Could you check a few things on this model? Use its own coordinates, in mm. A direction names the side the tool comes from. Coordinates: 2 decimals unless noted, no trailing zeros. Loops run counter-clockwise (first coordinate to the right, second up) from the corner with the lowest first, then second, coordinate; pieces in that order, holes last.
1) Imagine slicing it at C-C on y = 68. Please give me the cut outline in (x, z) (3 decimals), plus the area to 3 significant figures.
2) If I drill on line 1 along X through (y, z) = (61, 18.5) (3 decimals); line 2 along Z through (x, y) = (-19, 66.5); line 3 along Z through (x, y) = (-28, 26), over which ranges is the centre line in solid material (lowest first)?
3) Imagine slicing it at B-B on z = 1.5. Please give me the cut outline in (x, y), plus the area to 3 significant figures.
4) For faces 1 (the face through (-2, 38, 46.253)), 2 (the face through (-3.175, 38, 21)), which set-ups out of +Z, -Z, +X, -X, +Y, -Y let a thin tool reach every point of the face, with its end or its side?
5) Imagine slicing it at D-D on x = -25. Please give me the cut outline in (y, z).
6) Will these pins go through, and if not, where does the flat tip stop? P1, Ø12, axis at x = -7, z = -13.5, coming from the +Y side; P2, Ø21, axis at y = 41, z = 33.5, coming from the -X side (3 decimals); P3, Ø6, axis at y = 35.5, z = -15.5, coming from the -X side; P4, Ø1.5, axis at x = -32.5, y = 48.5, coming from the -Z side.
7) Imagine slicing it at A-A on y = 47.5. Please give me the cut outline in (x, z) (3 decimals), plus the area to 3 significant figures.
```python
from build123d import *

# Parameters (mm, degrees)
BOSS_EXTRUDE2_DEPTH = 76.2
CUT_EXTRUDE3_REACH  = 43.301
CUT_EXTRUDE4_REACH  = 62.908
FILLET1_R           = 5.08
FILLET2_R           = 3.81


with BuildPart() as part:
    # Sketch1 → Boss-Extrude2 (new body)
    with BuildSketch(Plane(origin=(0, 0, 0), x_dir=(1, 0, 0), z_dir=(0, 1, 0))):
        with BuildLine():
            Line((-39.668156778, 23.786852448), (-3.577868638, 2.145454699))
            ThreePointArc((-3.577868638, 2.145454699), (-0.956579917, -0.541770779), (0, -4.171824524))
            Line((0, -4.171824524), (0, -46.2534))
            Line((0, -46.2534), (-3.175, -46.2534))
            Line((-3.175, -46.2534), (-3.175, -4.171824524))
            ThreePointArc((-3.175, -4.171824524), (-3.719260987, -2.106449117), (-5.21068388, -0.577510483))
            Line((-5.21068388, -0.577510483), (-41.300972021, 21.063887265))
            Line((-41.300972021, 21.063887265), (-39.668156778, 23.786852448))
        make_face()
    extrude(amount=BOSS_EXTRUDE2_DEPTH)

    # Sketch2 → Cut-Extrude3 (cut, up to next)
    with BuildSketch(Plane(origin=(0, 0, 0), x_dir=(0, 0, -1), z_dir=(1, 0, 0)), mode=Mode.PRIVATE) as cut_extrude3_sk1:
        Polygon((-46.2534, 53.975), (-18.494383897, 76.2), (-46.2534, 76.2), align=None)
    cut_extrude3_tool1 = extrude(cut_extrude3_sk1.sketch, amount=-CUT_EXTRUDE3_REACH, mode=Mode.PRIVATE) & part.part
    add(cut_extrude3_tool1.solids().sort_by_distance((0, 68.791667, 37.000395))[0], mode=Mode.SUBTRACT)
    # Sketch2 → Cut-Extrude3 (cut, up to next)
    with BuildSketch(Plane(origin=(0, 0, 0), x_dir=(0, 0, -1), z_dir=(1, 0, 0)), mode=Mode.PRIVATE) as cut_extrude3_sk2:
        Polygon((-46.2534, 22.225), (-46.2534, 0), (-18.494383897, 0), align=None)
    cut_extrude3_tool2 = extrude(cut_extrude3_sk2.sketch, amount=-CUT_EXTRUDE3_REACH, mode=Mode.PRIVATE) & part.part
    add(cut_extrude3_tool2.solids().sort_by_distance((0, 7.408333, 37.000395))[0], mode=Mode.SUBTRACT)

    # Sketch4 → Cut-Extrude4 (cut, up to next)
    with BuildSketch(Plane(origin=(0, 0, 0), x_dir=(-0.857626829, 0, -0.514272517), z_dir=(0.514272517, 0, -0.857626829)), mode=Mode.PRIVATE) as cut_extrude4_sk1:
        Polygon((46.2534, 53.975), (18.494383897, 76.2), (46.2534, 76.2), align=None)
    cut_extrude4_tool1 = extrude(cut_extrude4_sk1.sketch, amount=-CUT_EXTRUDE4_REACH, mode=Mode.PRIVATE) & part.part
    add(cut_extrude4_tool1.solids().sort_by_distance((-31.732531, 68.791667, -19.028286))[0], mode=Mode.SUBTRACT)
    # Sketch4 → Cut-Extrude4 (cut, up to next)
    with BuildSketch(Plane(origin=(0, 0, 0), x_dir=(-0.857626829, 0, -0.514272517), z_dir=(0.514272517, 0, -0.857626829)), mode=Mode.PRIVATE) as cut_extrude4_sk2:
        Polygon((18.494383897, 0), (46.2534, 22.225), (46.2534, 0), align=None)
    cut_extrude4_tool2 = extrude(cut_extrude4_sk2.sketch, amount=-CUT_EXTRUDE4_REACH, mode=Mode.PRIVATE) & part.part
    add(cut_extrude4_tool2.solids().sort_by_distance((-31.732531, 7.408333, -19.028286))[0], mode=Mode.SUBTRACT)

    # Fillet1
    fillet1_edges = [part.edges().sort_by_distance(p)[0] for p in [
        (-1.5875, 22.225, 46.2534),
        (-1.5875, 53.975, 46.2534),
        (-40.4845644, 22.225, -22.425369856),
        (-40.4845644, 53.975, -22.425369856),
    ]]
    fillet(fillet1_edges, radius=FILLET1_R)

    # Fillet2
    fillet2_edges = [part.edges().sort_by_distance(p)[0] for p in [
        (-1.5875, 0, 18.494383897),
        (-1.5875, 76.2, 18.494383897),
        (-16.677687439, 0, -8.14967077),
        (-16.677687439, 76.2, -8.14967077),
    ]]
    fillet(fillet2_edges, radius=FILLET2_R)


solid = part.part
```
Filled in:
1. outline: (-26.278, -12.055) - (-24.645, -14.778) - (-3.578, -2.145) arc R7.366 ccw to (0, 4.172) - (0, 28.736) - (-3.175, 28.736) - (-3.175, 4.172) arc R4.191 cw to (-5.211, 0.578) - close
1. area: 175 mm2
2. line 1: x = -3.175 to 0
2. line 2: z = -11.39 to -7.69
2. line 3: z = -16.79 to -13.09
3. outline: (-4.14, 0) - (-0.5, 0) - (-0.5, 76.2) - (-4.14, 76.2) - close
3. area: 277 mm2
4. face 1: +Z, +X, -X, +Y, -Y
4. face 2: +Z, -X, +Y, -Y
5. outline: (7.01, -11.29) - (8.53, -14.99) - (67.67, -14.99) - (69.19, -11.29) - close
6. P1: passes through
6. P2: stops at x = -3.175
6. P3: stops at x = -37.03
6. P4: stops at z = -19.94
7. outline: (-41.301, -21.064) - (-39.668, -23.787) - (-3.578, -2.145) arc R7.366 ccw to (0, 4.172) - (0, 46.253) - (-3.175, 46.253) - (-3.175, 4.172) arc R4.191 cw to (-5.211, 0.578) - close
7. area: 286 mm2
